Geometry check sheet. Reference: the model listing, model coordinates, mm. Face numbers are marked on the shaded views. A direction names the side the tool comes from. Round coordinates to 2 decimals unless told otherwise and drop trailing zeros. Write each loop counter-clockwise with the first axis right and the second up, starting at its lowest first coordinate (ties: lowest second). Pieces come first, ordered by that corner, then holes.
Autodesk Inventor part; units mm, degrees
ref_plane "YZ Plane" through (0, 0, 0) normal (1, 0, 0) x (0, 1, 0)
ref_plane "XZ Plane" through (0, 0, 0) normal (0, 1, 0) x (-1, 0, 0)
ref_plane "XY Plane" through (0, 0, 0) normal (0, 0, 1) x (1, 0, 0)
sketch "Sketch1" plane through (0, 0, 0) normal (0, 0, 1) x (1, 0, 0)
  line L0 (0, 0) -> (0, 3.1469)
  line L1 (4.7625, 0) -> (4.7625, 3.937)
  line L2 (4.7625, 3.937) -> (5.55, 3.937)
  line L3 (5.55, 3.937) -> (5.55, 3.737)
  line L4 (5.55, 3.737) -> (5.65, 3.737)
  line L5 (5.65, 3.737) -> (5.65, 3.837)
  line L6 (5.65, 3.837) -> (7.05, 3.837)
  line L7 (7.05, 3.837) -> (7.05, 3.737)
  line L8 (7.05, 3.737) -> (7.15, 3.737)
  line L9 (7.15, 3.737) -> (7.15, 3.937)
  line L10 (7.15, 3.937) -> (7.9375, 3.937)
  line L11 (7.9375, 3.937) -> (7.9375, 0)
  line L12 (7.9375, 0) -> (7.15, 0)
  line L13 (7.15, 0) -> (7.15, 0.25)
  line L14 (7.15, 0.25) -> (7.05, 0.25)
  line L15 (7.05, 0.25) -> (7.05, 0.1)
  line L16 (7.05, 0.1) -> (5.65, 0.1)
  line L17 (5.65, 0.1) -> (5.65, 0.25)
  line L18 (5.65, 0.25) -> (5.55, 0.25)
  line L19 (5.55, 0.25) -> (5.55, 0)
  line L20 (5.55, 0) -> (4.7625, 0)
  line L21 (4.7625, 1.9685) -> (7.9375, 1.9685) construction
  point P0 (6.35, 0.1)
  point P1 (6.35, 1.9685)
  dimension "d0" = 9.525
  dimension "d1" = 3.937
  dimension "d2" = 15.875
  dimension "d3" = 0.1
  dimension "d4" = 0.25
  dimension "d5" = 0.1
  dimension "d6" = 0.1
  dimension "d7" = 1.4
  dimension "d8" = 0.2
revolve "Revolution1" add sketch "Sketch1" angle 360 about axis through (0, 0, 0) along (0, 1, 0)
chamfer "Chamfer1" distance 0.35 angle 45 4 edges at (-4.7625, 3.937, 0) (-7.9375, 3.937, 0) (-7.9375, 0, 0) (-4.7625, 0, 0)
properties part number "R1038_ZZ_W Bearing" material "Stainless Steel"
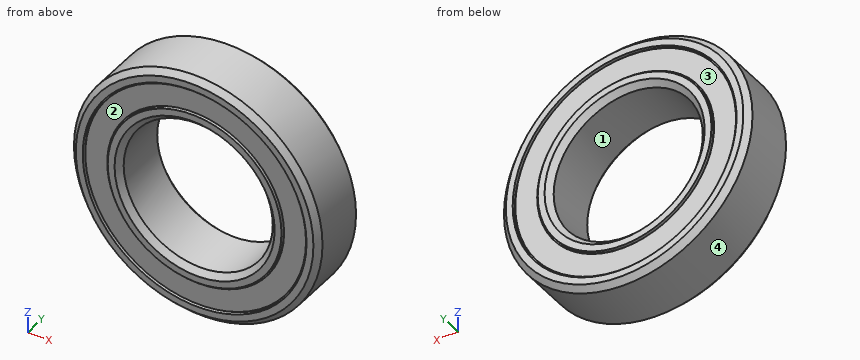
1. Scan lines: line 1 along Z through (x, y) = (0, 1.5); line 2 along Y through (x, z) = (-2.75, 6.25). Record each from-to range of solid material in increasing order.
2. Access from +Z, -Z, +X, -X, +Y, -Y to the whole of each face (thin tool, end or side, straight path). Record for the marked faces 1 and 2.
3. Depth check by flat-ended pin: pin 1 Ø4 at (x, z) = (0, 3) entering from -Y. Enter the tip coordinate at first touch or a pass-through.
4. Release check for a two-part mould opening along X. For the marked faces 3 and 4 record: +X half, -X half, draft (parallel to the pull), parting line (faces both ways), or undercut.
5. Section check A-A (y = 2.1). Record the cut outline in (x, z) (1 decimal), plus the area to 3 significant figures.
Results below:
1. line 1: z = -7.94 to -4.76, 4.76 to 7.94
1. line 2: y = 0.1 to 3.84
2. face 1: +Y, -Y
2. face 2: -Y
3. pin 1: stops at y = 0.11
4. face 3: undercut
4. face 4: parting line
5. outline: circle Ø15.9 at (0, 0); hole circle Ø9.5 at (0, 0)
5. area: 127 mm2
